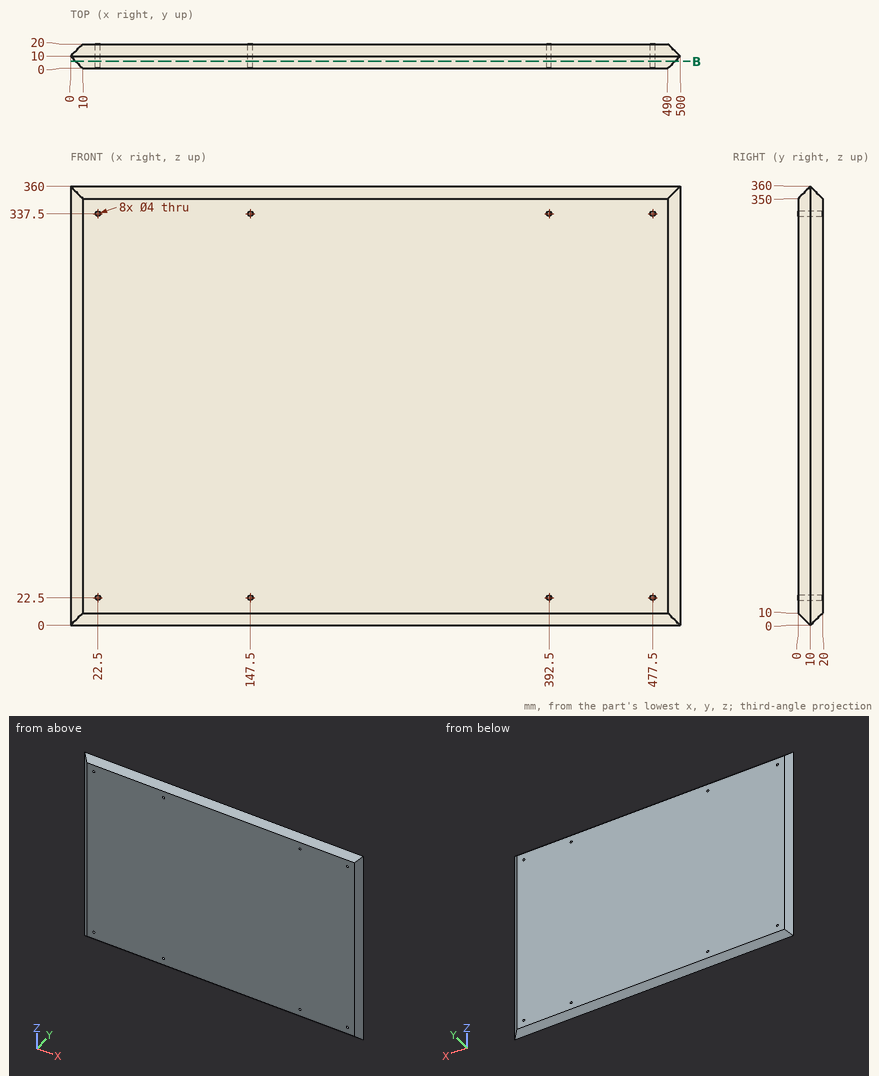
Answer from the drawing. Dimensions are ordinates in mm from the lowest x, y and z of the part. Coordinates: 2 decimals unless noted, no trailing zeros. Write item = value, one per line.
1. Straight lines are drawn through the part: line 1 (Z direction, x = 22.5, y = 6); line 2 (X direction, y = 7.5, z = 22.5); line 3 (X direction, y = 8.5, z = 22.5). For each, find the intervals that lie inside material, in ascending order. Write a range as from..to.
Solution:
line_1 = 4..20.5, 24.5..335.5, 339.5..356
line_2 = 2.5..20.5, 24.5..145.5, 149.5..390.5, 394.5..475.5, 479.5..497.5
line_3 = 1.5..20.5, 24.5..145.5, 149.5..390.5, 394.5..475.5, 479.5..498.5
2. The part is cut by section B-B (y = 5.75). State how many separate pieces and enclosed holes the cut face has, then the cut area to 3 significant figures.
Solution:
separate_pieces = 1
enclosed_holes = 8
area = 173,000 mm2
3. Flat-ended cylindrical pins translate along their axes: pin 1 (2 mm diameter, centred on x = 180.5, y = 14.5, fed in from -Z); pin 2 (4 mm diameter, centred on x = 272, y = 16, fed in from +Z); pin 3 (3 mm diameter, centred on y = 17.5, z = 203.5, fed in from +X); pin 4 (2.5 mm diameter, centred on x = 147.5, z = 22.5, fed in from -Y). Find the tip coordinate at first contact, or state that the pin passes through.
Solution:
pin_1 = 3.5
pin_2 = 356
pin_3 = 494
pin_4 = through
